Check sheet for the modelled part. Datum: model origin and axes. Units: mm. A direction names the side the tool comes from. Give positions to 0.01 mm unless a question says otherwise; leave off trailing zeros. Order: outer loops, then holes, each group sorted by start corner. A loop starts at its lowest first (then second) coordinate and runs counter-clockwise, first axis right, second up. Notation, with made-up numbers: (-26.5, 41.5) - (32.5, 41.5) arc R24 ccw to (32.5, 80.5) - close; hole circle Ø9 at (-34, -7.5). An arc over 180 degrees is marked (long way). Answer in a Markdown table with one row per item.
from build123d import *

# Parameters (mm, degrees)
ESQUISSE1_W        = 90
ESQUISSE1_H        = 20
ESQUISSE1_W_2      = 250
BOSS_EXTRU_1_DEPTH = 5
BOSS_EXTRU_2_DEPTH = 250


with BuildPart() as part:
    # Esquisse1 → Boss.-Extru.1 (new body)
    with BuildSketch(Plane.XY):
        with Locations((-125, 30)):
            Rectangle(ESQUISSE1_W, ESQUISSE1_H)
        with Locations((-125, 10)):
            Rectangle(ESQUISSE1_W_2, ESQUISSE1_H)
    extrude(amount=BOSS_EXTRU_1_DEPTH)

    # Esquisse2 → Boss.-Extru.2 (add)
    with BuildSketch(Plane(origin=(0, 0, 0), x_dir=(0, 0, -1), z_dir=(1, 0, 0))):
        Polygon((-25, 0), (-5, 0), (-5, 5), (-10, 5), align=None)
    extrude(amount=-BOSS_EXTRU_2_DEPTH)


solid = part.part
(1) Cross-section at C-C, the plane y = 35. Record the cut outline in (x, z).
Geometry says:
| item | result |
|---|---|
| outline | (-170, 0) - (-80, 0) - (-80, 5) - (-170, 5) - close |
(2) Gauge pin test, flat ends, axial feed: P1, Ø6, axis at x = -224.5, z = 6, coming from the +Y side; P2, Ø2, axis at x = -30.5, z = 20, coming from the +Y side; P3, Ø12, axis at x = -108, z = 8, coming from the -Y side; P4, Ø1.5, axis at y = 29, z = 2, coming from the -X side. Record the tip position at first contact, or that the pin passes through.
Geometry says:
| item | result |
|---|---|
| P1 | y = 20 |
| P2 | y = 2 |
| P3 | y = 0 |
| P4 | x = -170 |
(3) Thickness scan on L1, parallel to Z at x = -117.5, y = 37.5; L2, parallel to Y at x = -208, z = 3.75; L3, parallel to X at y = 27, z = 1.75. Record the ranges inside material, lowest first.
Geometry says:
| item | result |
|---|---|
| L1 | 0 to 5 |
| L2 | 0 to 20 |
| L3 | -170 to -80 |
(4) Cross-section at A-A, the plane x = -129.5. Record the cut outline in (y, z).
Geometry says:
| item | result |
|---|---|
| outline | (0, 0) - (40, 0) - (40, 5) - (5, 5) - (5, 10) - (0, 25) - close |
(5) Access from +Z, -Z, +X, -X, +Y, -Y to the whole of each face (thin tool, end or side, straight path). Record for faces 1 (the flat face through (-127, 19, 5)), 2 (the flat face through (-80, 30, 2)), 3 (the flat face through (-170, 30, 2)).
Geometry says:
| item | result |
|---|---|
| face 1 | +Z, +X, -X, +Y |
| face 2 | +Z, -Z, +X, +Y |
| face 3 | +Z, -Z, -X, +Y |
(6) Cross-section at D-D, the plane x = -45. Record the cut outline in (y, z).
Geometry says:
| item | result |
|---|---|
| outline | (0, 0) - (20, 0) - (20, 5) - (5, 5) - (5, 10) - (0, 25) - close |
(7) Cross-section at B-B, the plane z = 2.75. Record the cut outline in (x, y).
Geometry says:
| item | result |
|---|---|
| outline | (-250, 0) - (0, 0) - (0, 20) - (-80, 20) - (-80, 40) - (-170, 40) - (-170, 20) - (-250, 20) - close |
